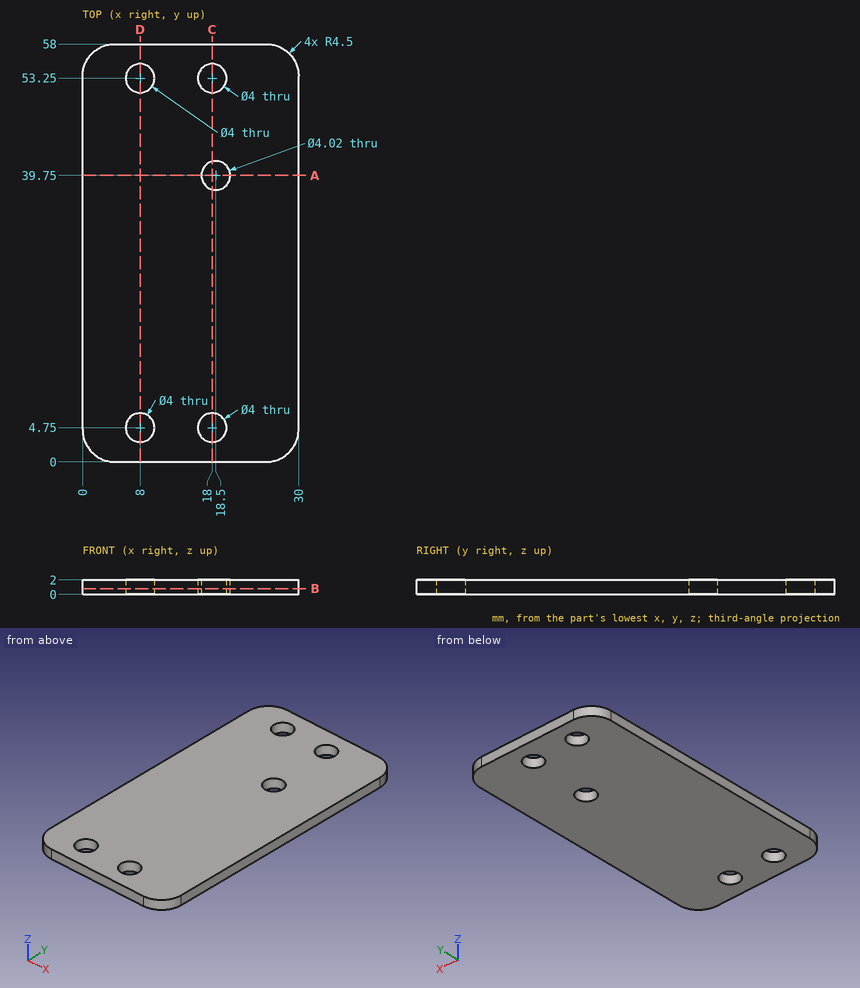
Drawing for the job (mm, zero at the part's lowest x, y, z). Coordinates: 2 decimals unless noted, no trailing zeros. Order: outer loops, then holes, each group sorted by start corner. A loop starts at its lowest first (then second) coordinate and runs counter-clockwise, first axis right, second up. Notation, with made-up numbers: (41.5, 39) - (71.5, 39) arc R10 ccw to (71.5, 48) - close; hole circle Ø7 at (74, 54.25). An arc over 180 degrees is marked (long way). Use a Markdown table: item, result. Add a question column.
(1) Flat gauge pins, fed straight in: pin 1 (6.5 mm diameter, centred on x = 8, y = 4.75, fed in from -Z); pin 2 (3 mm diameter, centred on x = 18.5, y = 39.75, fed in from +Z). Where does each tip first touch, or does it go through?
(2) Saw through at B-B (z = 0.8). Give the cut face in (x, y).
(3) Saw through at A-A (y = 39.75). Give the cut face in (x, z), then the cut area to 3 significant figures.
(4) Saw through at C-C (x = 18). Give the cut face in (y, z).
(5) Drill centre lines: line 1 along Y through (x, z) = (18.5, 1.55); line 2 along Y through (x, z) = (18, 0.7); line 3 along Y through (x, z) = (7.5, 1.25). Where is each one in solid material? Low to high. Write a range as [from, to].
(6) Saw through at D-D (x = 8). Give the cut face in (y, z), then the cut area to 3 significant figures.
Solved:
| question | item | result |
|---|---|---|
| 1 | pin 1 | stops at z = 0 |
| 1 | pin 2 | passes through |
| 2 | outline | (0, 4.5) arc R4.5 ccw to (4.5, 0) - (25.5, 0) arc R4.5 ccw to (30, 4.5) - (30, 53.5) arc R4.5 ccw to (25.5, 58) - (4.5, 58) arc R4.5 ccw to (0, 53.5) - close; hole circle Ø4 at (8, 4.75); hole circle Ø4 at (8, 53.25); hole circle Ø4 at (18, 4.75); hole circle Ø4 at (18, 53.25); hole circle Ø4.02 at (18.5, 39.75) |
| 3 | outline | (0, 0) - (16.49, 0) - (16.49, 2) - (0, 2) - close; (20.51, 0) - (30, 0) - (30, 2) - (20.51, 2) - close |
| 3 | area | 52.0 mm² |
| 4 | outline | (0, 0) - (2.75, 0) - (2.75, 2) - (0, 2) - close; (6.75, 0) - (37.8, 0) - (37.8, 2) - (6.75, 2) - close; (41.7, 0) - (51.25, 0) - (51.25, 2) - (41.7, 2) - close; (55.25, 0) - (58, 0) - (58, 2) - (55.25, 2) - close |
| 5 | line 1 | y = [0, 2.81], [6.69, 37.74], [41.76, 51.31], [55.19, 58] |
| 5 | line 2 | y = [0, 2.75], [6.75, 37.8], [41.7, 51.25], [55.25, 58] |
| 5 | line 3 | y = [0, 2.81], [6.69, 51.31], [55.19, 58] |
| 6 | outline | (0, 0) - (2.75, 0) - (2.75, 2) - (0, 2) - close; (6.75, 0) - (51.25, 0) - (51.25, 2) - (6.75, 2) - close; (55.25, 0) - (58, 0) - (58, 2) - (55.25, 2) - close |
| 6 | area | 100 mm² |
